Part model, mm, in its own coordinate system. A direction names the side the tool comes from. Give positions to 0.01 mm unless a question says otherwise; leave off trailing zeros. Order: outer loops, then holes, each group sorted by start corner. A loop starts at its lowest first (then second) coordinate and runs counter-clockwise, first axis right, second up.
1. Slice it at A-A on x = -24. List the corners of the cut face in (y, z), and give its area (3 significant figures).
2. Which spindle directions (+Z, -Z, +X, -X, +Y, -Y) get a long thin tool onto all of the face, cutting with end or side? Do faces 4 (the flat face through (30, 50, -2)), 5 (the flat face through (48, 52, 5)), 6 (the flat face through (-26, -52, 5)), 7 (the cylindrical face through (-56, -46.07, 5.07)). Say none if no direction does.
3. Probe line 1 (X direction, y = -53, z = -2.5); line 2 (Y direction, x = 37, z = 10.5); line 3 (Y direction, x = 13.35, z = 4.5). List the from-to ranges inside material, lowest first.
4. Slice it at B-B on y = 25. List the corners of the cut face in (x, z).
5. Mould opens along Y. For faces 1 (the cylindrical face through (12.479, -55.854, -2.704)), 2 (the flat face through (-57.5, -1, 5)), 3 (the flat face through (-14, -55, 4)) say: +Y half, -Y half, draft (parallel to the pull), parting line (faces both ways), or undercut.
6. Drop flat-ended pins along their axis: pin 1 Ø3.5 at (y, z) = (-57, 4.5) entering from +X; pin 2 Ø0.8 at (x, z) = (-11.5, 10.5) entering from -Y; pin 3 Ø6 at (x, y) = (-42, 30) entering from +Z. Give the stop position or say it passes through.
from build123d import *

# Parameters (mm, degrees)
SKETCH1_W            = 124
SKETCH1_H            = 104
SKETCH1_W_2          = 115
SKETCH1_H_2          = 95
BOSS_EXTRUDE1_DEPTH  = 10
SKETCH1_2_W          = 124
SKETCH1_2_H          = 104
BOSS_EXTRUDE2_DEPTH  = 3
FILLET1_R            = 8.25
FILLET2_R            = 5
BOSS_EXTRUDE3_DEPTH  = 1
CHAMFER1_SIZE        = 3
BOSS_EXTRUDE4_START  = -24.8
SKETCH3_R            = 1.6
BOSS_EXTRUDE4_DEPTH  = 6
BOSS_EXTRUDE5_START  = -105.2
SKETCH3_4_R          = 1.6
BOSS_EXTRUDE5_DEPTH  = 6
BOSS_EXTRUDE6_START  = -45.7
SKETCH3_6_R          = 1.4
BOSS_EXTRUDE6_DEPTH  = 6
BOSS_EXTRUDE7_START  = -84.3
SKETCH3_7_R          = 1.4
BOSS_EXTRUDE7_DEPTH  = 6
FILLET3_R            = 2
FILLET4_R            = 5
BOSS_EXTRUDE8_START  = -25
BOSS_EXTRUDE8_DEPTH  = 3
BOSS_EXTRUDE9_START  = -96
SKETCH4_3_R          = 1.6
BOSS_EXTRUDE9_DEPTH  = 3
BOSS_EXTRUDE10_START = -48
BOSS_EXTRUDE10_DEPTH = 3
BOSS_EXTRUDE11_START = -76
SKETCH4_6_R          = 1.4
BOSS_EXTRUDE11_DEPTH = 3
CHAMFER2_SIZE        = 6
FILLET5_R            = 5
FILLET6_R            = 2
FILLET7_R            = 1
FILLET8_R            = 4


with BuildPart() as part:
    # Sketch1 → Boss-Extrude1 (new body)
    with BuildSketch(Plane.XY):
        Rectangle(SKETCH1_W, SKETCH1_H)
        Rectangle(SKETCH1_W_2, SKETCH1_H_2, mode=Mode.SUBTRACT)
    extrude(amount=BOSS_EXTRUDE1_DEPTH)

    # Sketch1_2 → Boss-Extrude2 (add)
    with BuildSketch(Plane.XY):
        Rectangle(SKETCH1_2_W, SKETCH1_2_H)
    extrude(amount=-BOSS_EXTRUDE2_DEPTH)

    # Fillet1
    fillet1_edges = [part.edges().sort_by_distance(p)[0] for p in [
        (-62, 52, 3.5),
        (62, 52, 3.5),
        (62, -52, 3.5),
        (-62, -52, 3.5),
    ]]
    fillet(fillet1_edges, radius=FILLET1_R)

    # Fillet2
    fillet2_edges = [part.edges().sort_by_distance(p)[0] for p in [
        (-57.5, 47.5, 5),
        (-57.5, -47.5, 5),
        (57.5, -47.5, 5),
        (57.5, 47.5, 5),
    ]]
    fillet(fillet2_edges, radius=FILLET2_R)

    # Sketch2 → Boss-Extrude3 (add)
    with BuildSketch(Plane.XY.offset(10)):
        with BuildLine():
            ThreePointArc((52.5, 50.25), (57.980077554, 47.980077554), (60.25, 42.5))
            Line((60.25, 42.5), (60.25, -42.5))
            ThreePointArc((60.25, -42.5), (57.980077554, -47.980077554), (52.5, -50.25))
            Line((52.5, -50.25), (-52.5, -50.25))
            ThreePointArc((-52.5, -50.25), (-57.980077554, -47.980077554), (-60.25, -42.5))
            Line((-60.25, -42.5), (-60.25, 42.5))
            ThreePointArc((-60.25, 42.5), (-57.980077554, 47.980077554), (-52.5, 50.25))
            Line((-52.5, 50.25), (52.5, 50.25))
        make_face()
        with BuildLine():
            ThreePointArc((52.5, -49.25), (57.272970773, -47.272970773), (59.25, -42.5))
            Line((59.25, -42.5), (59.25, 42.5))
            ThreePointArc((59.25, 42.5), (57.272970773, 47.272970773), (52.5, 49.25))
            Line((52.5, 49.25), (-52.5, 49.25))
            ThreePointArc((-52.5, 49.25), (-57.272970773, 47.272970773), (-59.25, 42.5))
            Line((-59.25, 42.5), (-59.25, -42.5))
            ThreePointArc((-59.25, -42.5), (-57.272970773, -47.272970773), (-52.5, -49.25))
            Line((-52.5, -49.25), (52.5, -49.25))
        make_face(mode=Mode.SUBTRACT)
    extrude(amount=BOSS_EXTRUDE3_DEPTH)

    # Chamfer1
    chamfer1_edges = [part.edges().sort_by_distance(p)[0] for p in [
        (0, 52, -3),
        (62, 0, -3),
        (0, -52, -3),
        (-62, 0, -3),
        (-59.583630945, 49.583630945, -3),
        (-59.583630945, -49.583630945, -3),
        (59.583630945, -49.583630945, -3),
        (59.583630945, 49.583630945, -3),
    ]]
    chamfer(chamfer1_edges, length=CHAMFER1_SIZE)

    # Sketch3 → Boss-Extrude4 (add)
    with BuildSketch(Plane.ZY.offset(62).offset(BOSS_EXTRUDE4_START)):
        with BuildLine():
            ThreePointArc((10, 52), (13.092758443, 56.248671724), (8.099292057, 57.8862491))
            Line((8.099292057, 57.8862491), (2.015640289, 53.5))
            Line((2.015640289, 53.5), (-3, 53.5))
            Line((-3, 53.5), (-3, 49))
            Line((-3, 49), (0, 52))
            Line((0, 52), (10, 52))
        make_face()
        with Locations(Location((10, 55.25, 0), (0, 0, 270))):
            Circle(SKETCH3_R, mode=Mode.SUBTRACT)
    extrude(amount=BOSS_EXTRUDE4_DEPTH)

    # Sketch3_4 → Boss-Extrude5 (add)
    with BuildSketch(Plane.ZY.offset(62).offset(BOSS_EXTRUDE5_START)):
        with BuildLine():
            ThreePointArc((10, 52), (13.092758443, 56.248671724), (8.099292057, 57.8862491))
            Line((8.099292057, 57.8862491), (2.015640289, 53.5))
            Line((2.015640289, 53.5), (-3, 53.5))
            Line((-3, 53.5), (-3, 49))
            Line((-3, 49), (0, 52))
            Line((0, 52), (10, 52))
        make_face()
        with Locations(Location((10, 55.25, 0), (0, 0, 270))):
            Circle(SKETCH3_4_R, mode=Mode.SUBTRACT)
    extrude(amount=BOSS_EXTRUDE5_DEPTH)

    # Sketch3_6 → Boss-Extrude6 (add)
    with BuildSketch(Plane.ZY.offset(62).offset(BOSS_EXTRUDE6_START)):
        with BuildLine():
            ThreePointArc((10, 52), (13.092758443, 56.248671724), (8.099292057, 57.8862491))
            Line((8.099292057, 57.8862491), (2.015640289, 53.5))
            Line((2.015640289, 53.5), (-3, 53.5))
            Line((-3, 53.5), (-3, 49))
            Line((-3, 49), (0, 52))
            Line((0, 52), (10, 52))
        make_face()
        with Locations(Location((10, 55.25, 0), (0, 0, 270))):
            Circle(SKETCH3_6_R, mode=Mode.SUBTRACT)
    extrude(amount=BOSS_EXTRUDE6_DEPTH)

    # Sketch3_7 → Boss-Extrude7 (add)
    with BuildSketch(Plane.ZY.offset(62).offset(BOSS_EXTRUDE7_START)):
        with BuildLine():
            ThreePointArc((10, 52), (13.092758443, 56.248671724), (8.099292057, 57.8862491))
            Line((8.099292057, 57.8862491), (2.015640289, 53.5))
            Line((2.015640289, 53.5), (-3, 53.5))
            Line((-3, 53.5), (-3, 49))
            Line((-3, 49), (0, 52))
            Line((0, 52), (10, 52))
        make_face()
        with Locations(Location((10, 55.25, 0), (0, 0, 270))):
            Circle(SKETCH3_7_R, mode=Mode.SUBTRACT)
    extrude(amount=BOSS_EXTRUDE7_DEPTH)

    # Fillet3
    fillet3_edges = [part.edges().sort_by_distance(p)[0] for p in [
        (-40.2, 53.5, -3),
        (40.2, 53.5, -3),
        (-19.3, 53.5, -3),
        (19.3, 53.5, -3),
    ]]
    fillet(fillet3_edges, radius=FILLET3_R)

    # Fillet4
    fillet4_edges = [part.edges().sort_by_distance(p)[0] for p in [
        (-40.2, 53.5, 2.015640289),
        (40.2, 53.5, 2.015640289),
        (-19.3, 53.5, 2.015640289),
        (19.3, 53.5, 2.015640289),
    ]]
    fillet(fillet4_edges, radius=FILLET4_R)

    # Sketch4 → Boss-Extrude8 (add)
    with BuildSketch(Plane(origin=(62, 0, 0), x_dir=(0, 0, -1), z_dir=(1, 0, 0)).offset(BOSS_EXTRUDE8_START)):
        with BuildLine():
            Line((3, -57), (3, -49))
            Line((3, -49), (0, -52))
            Line((0, -52), (-10, -52))
            Line((-10, -52), (-10, -57))
            Line((-10, -57), (-6.1, -57))
            ThreePointArc((-6.1, -57), (-4.5, -55.4), (-2.9, -57))
            Line((-2.9, -57), (3, -57))
        make_face()
        with BuildLine():
            Line((3, -62), (3, -57))
            Line((3, -57), (-2.9, -57))
            ThreePointArc((-2.9, -57), (-4.5, -58.6), (-6.1, -57))
            Line((-6.1, -57), (-10, -57))
            Line((-10, -57), (-10, -62))
            Line((-10, -62), (3, -62))
        make_face()
    extrude(amount=-BOSS_EXTRUDE8_DEPTH)

    # Sketch4_3 → Boss-Extrude9 (add)
    with BuildSketch(Plane(origin=(62, 0, 0), x_dir=(0, 0, -1), z_dir=(1, 0, 0)).offset(BOSS_EXTRUDE9_START)):
        Polygon((3, -62), (3, -49), (0, -52), (-10, -52), (-10, -62), align=None)
        with Locations(Location((-4.5, -57, 0), (0, 0, 90))):
            Circle(SKETCH4_3_R, mode=Mode.SUBTRACT)
    extrude(amount=-BOSS_EXTRUDE9_DEPTH)

    # Sketch4_5 → Boss-Extrude10 (add)
    with BuildSketch(Plane(origin=(62, 0, 0), x_dir=(0, 0, -1), z_dir=(1, 0, 0)).offset(BOSS_EXTRUDE10_START)):
        with BuildLine():
            Line((3, -57), (3, -49))
            Line((3, -49), (0, -52))
            Line((0, -52), (-10, -52))
            Line((-10, -52), (-10, -57))
            Line((-10, -57), (-6.1, -57))
            ThreePointArc((-6.1, -57), (-4.5, -55.4), (-2.9, -57))
            Line((-2.9, -57), (3, -57))
        make_face()
        with BuildLine():
            Line((3, -62), (3, -57))
            Line((3, -57), (-2.9, -57))
            ThreePointArc((-2.9, -57), (-4.5, -58.6), (-6.1, -57))
            Line((-6.1, -57), (-10, -57))
            Line((-10, -57), (-10, -62))
            Line((-10, -62), (3, -62))
        make_face()
        with BuildLine():
            ThreePointArc((-6.1, -57), (-4.5, -58.6), (-2.9, -57))
            Line((-2.9, -57), (-3.1, -57))
            ThreePointArc((-3.1, -57), (-4.5, -58.4), (-5.9, -57))
            Line((-5.9, -57), (-6.1, -57))
        make_face()
        with BuildLine():
            Line((-3.1, -57), (-2.9, -57))
            ThreePointArc((-2.9, -57), (-4.5, -55.4), (-6.1, -57))
            Line((-6.1, -57), (-5.9, -57))
            ThreePointArc((-5.9, -57), (-4.5, -55.6), (-3.1, -57))
        make_face()
    extrude(amount=-BOSS_EXTRUDE10_DEPTH)

    # Sketch4_6 → Boss-Extrude11 (add)
    with BuildSketch(Plane(origin=(62, 0, 0), x_dir=(0, 0, -1), z_dir=(1, 0, 0)).offset(BOSS_EXTRUDE11_START)):
        Polygon((3, -62), (3, -49), (0, -52), (-10, -52), (-10, -62), align=None)
        with Locations(Location((-4.5, -57, 0), (0, 0, 90))):
            Circle(SKETCH4_6_R, mode=Mode.SUBTRACT)
    extrude(amount=-BOSS_EXTRUDE11_DEPTH)

    # Chamfer2
    chamfer2_edges = [part.edges().sort_by_distance(p)[0] for p in [
        (35.5, -62, -3),
        (-35.5, -62, -3),
        (12.5, -62, -3),
        (-15.5, -62, -3),
    ]]
    chamfer(chamfer2_edges, length=CHAMFER2_SIZE)

    # Fillet5
    fillet5_edges = [part.edges().sort_by_distance(p)[0] for p in [
        (35.5, -62, 10),
        (-35.5, -62, 10),
        (12.5, -62, 10),
        (-15.5, -62, 10),
    ]]
    fillet(fillet5_edges, radius=FILLET5_R)

    # Fillet6
    fillet6_edges = [part.edges().sort_by_distance(p)[0] for p in [
        (-35.5, -62, 3),
        (-15.5, -62, 3),
        (12.5, -62, 3),
        (35.5, -62, 3),
    ]]
    fillet(fillet6_edges, radius=FILLET6_R)

    # Fillet7
    fillet7_edges = [part.edges().sort_by_distance(p)[0] for p in [
        (34, -52, 5),
        (34, -50.5, -1.5),
        (37, -50.5, -1.5),
        (37, -52, 5),
        (-37, -50.5, -1.5),
        (-37, -52, 5),
        (-34, -50.5, -1.5),
        (-34, -52, 5),
        (11, -52, 5),
        (11, -50.5, -1.5),
        (14, -50.5, -1.5),
        (14, -52, 5),
        (-17, -50.5, -1.5),
        (-17, -52, 5),
        (-14, -50.5, -1.5),
        (-14, -52, 5),
    ]]
    fillet(fillet7_edges, radius=FILLET7_R)

    # Fillet8
    fillet8_edges = [part.edges().sort_by_distance(p)[0] for p in [
        (35.5, -56, -3),
        (12.5, -56, -3),
        (-15.5, -56, -3),
        (-35.5, -56, -3),
    ]]
    fillet(fillet8_edges, radius=FILLET8_R)


solid = part.part
Data:
1. outline: (-52, 0) - (-49, -3) - (49, -3) - (52, 0) - (52, 10) - (50.25, 10) - (50.25, 11) - (49.25, 11) - (49.25, 10) - (47.5, 10) - (47.5, 0) - (-47.5, 0) - (-47.5, 10) - (-49.25, 10) - (-49.25, 11) - (-50.25, 11) - (-50.25, 10) - (-52, 10) - close
1. area: 395 mm2
2. face 4: -Z, +Y
2. face 5: +Z, -Z, +X, +Y
2. face 6: +Z, -Z, -Y
2. face 7: +Z
3. line 1: x = -37 to -34, -17 to -14, 11 to 14, 34 to 37
3. line 2: y = -50.25 to -49.25, 49.25 to 50.25
3. line 3: y = -62 to -58.4, -55.6 to -47.5, 47.5 to 52
4. outline: (-62, 0) - (-59, -3) - (59, -3) - (62, 0) - (62, 10) - (60.25, 10) - (60.25, 11) - (59.25, 11) - (59.25, 10) - (57.5, 10) - (57.5, 0) - (-57.5, 0) - (-57.5, 10) - (-59.25, 10) - (-59.25, 11) - (-60.25, 11) - (-60.25, 10) - (-62, 10) - close
5. face 1: -Y half
5. face 2: undercut
5. face 3: draft
6. pin 1: stops at x = 37
6. pin 2: stops at y = -50.25
6. pin 3: stops at z = 0
